Autodesk Inventor part; units mm, degrees
ref_plane "YZ Plane" through (0, 0, 0) normal (1, 0, 0) x (0, 1, 0)
ref_plane "XZ Plane" through (0, 0, 0) normal (0, 1, 0) x (-1, 0, 0)
ref_plane "XY Plane" through (0, 0, 0) normal (0, 0, 1) x (1, 0, 0)
sketch "Sketch2" plane through (0, 0, 0) normal (0, 1, 0) x (-1, 0, 0)
  line L0 (-22.05, -28.75) -> (22.05, -28.75)
  line L1 (22.05, -28.75) -> (22.05, 28.75)
  line L2 (22.05, 28.75) -> (-22.05, 28.75)
  line L3 (-22.05, 28.75) -> (-22.05, -28.75)
  line L4 (-22.05, -28.75) -> (22.05, 28.75) construction
  line L5 (22.05, -28.75) -> (-22.05, 28.75) construction
  point P0 (0, 0)
  dimension "d28" = 44.1
  dimension "d29" = 57.5
extrude "Extrusion2" add sketch "Sketch2" along normal blind 0.5
sketch "Sketch3" plane through (0, 0.5, 0) normal (0, 1, 0) x (1, 0, 0)
  line L0 (3.17, 0) -> (-3.4256, 0) construction
  line L1 (-18, -28.75) -> (-18, -19.75)
  line L2 (-15.5, -19.75) -> (-15.5, -28.75)
  arc A0 (-15.5, -19.75) -> (-18, -19.75) centre (-16.75, -19.75) ccw
  line L3 (-22.05, -28.75) -> (22.05, -28.75)
  line L4 (-22.05, 28.75) -> (-22.05, -28.75)
  line L5 (19.8, -28.75) -> (19.8, -19.75)
  line L6 (17.3, -19.75) -> (17.3, -28.75)
  arc A1 (19.8, -19.75) -> (17.3, -19.75) centre (18.55, -19.75) ccw
  line L7 (15.5, 28.75) -> (15.5, 19.75)
  line L8 (22.05, 28.75) -> (-22.05, 28.75)
  line L9 (18, 28.75) -> (18, 19.75)
  arc A2 (15.5, 19.75) -> (18, 19.75) centre (16.75, 19.75) ccw
  line L10 (22.05, -28.75) -> (22.05, 28.75)
  line L11 (-19.8, 28.75) -> (-19.8, 19.75)
  line L12 (-17.3, 28.75) -> (-17.3, 19.75)
  arc A3 (-19.8, 19.75) -> (-17.3, 19.75) centre (-18.55, 19.75) ccw
  point P0 (0, 0)
  point P1 (10.634, -28.75)
  point P2 (12.3949, -28.75)
  dimension "d32" = 2.5
  dimension "d33" = 9
  dimension "d34" = 1.25
  dimension "d48" = 5.3
  dimension "d60" = 9
  dimension "d61" = 9
  dimension "d62" = 1.25
  dimension "d64" = 9
  dimension "d65" = 9
  dimension "d66" = 1.25
  dimension "d71" = 3.5
  dimension "d87" = 5.3
  dimension "d88" = 3.5
extrude "Extrusion3" cut sketch "Sketch3" against normal through all contours L1 A0 L2 L3 | L6 A1 L5 L3 | L8 L12 A3 L11 | L8 L9 A2 L7
sketch "Sketch4" plane through (0, 0.5, 0) normal (0, 1, 0) x (1, 0, 0)
  line L0 (-22.05, 28.75) -> (-22.05, -28.75)
  line L1 (-22.05, -28.75) -> (22.05, -28.75)
  line L2 (22.05, -28.75) -> (22.05, 28.75)
  line L3 (22.05, 28.75) -> (-22.05, 28.75)
  point P0 (0, 0)
  point P1 (0, -27.15)
  point P2 (0, 27.15)
  point P3 (-18, -28.75)
  point P4 (-12.775, 28.75)
  dimension "d37" = 22.05
  dimension "d38" = 1.6
  dimension "d40" = 1.6
  dimension "d68" = 44.1
hole "Hole1" at (0, 0.5, 27.15) at (0, 0.5, -27.15) direction (0, -1, 0) diameter 2.4 end through all
sketch "Sketch5" plane through (0, 0.5, 0) normal (0, 1, 0) x (1, 0, 0)
  line L0 (-22.05, -28.75) -> (-18, -28.75)
  line L1 (-20.05, -28.75) -> (-22.05, -26.75)
  line L2 (-22.05, 28.75) -> (-22.05, -28.75)
  point P0 (0, 0)
  dimension "d49" = 2
  dimension "d50" = 2
extrude "Extrusion4" cut sketch "Sketch5" against normal through all
sketch "Sketch6" plane through (0, 0.5, 0) normal (0, 1, 0) x (1, 0, 0)
  circle A0 centre (0, -27.15) radius 1.2
  line L0 (-1.2, -27.15) -> (-1.2, -28.75)
  line L1 (-15.5, -28.75) -> (17.3, -28.75)
  line L2 (1.2, -27.15) -> (1.2, -28.75)
  line L3 (1.2, -27.15) -> (-1.2, -27.15)
  line L4 (24.0299, 0) -> (-42.1887, 0)
  line L5 (-1.2, 27.15) -> (-1.2, 28.75)
  line L6 (1.2, 27.15) -> (1.2, 28.75)
  line L7 (1.2, 27.15) -> (-1.2, 27.15)
  line L8 (15.5, 28.75) -> (-17.3, 28.75)
  point P0 (0, 0)
  point P1 (0, 27.15)
extrude "Extrusion5" cut sketch "Sketch6" against normal through all contours L2 L1 L0 A0 | L5 L8 L6 L7
sketch "Sketch7" plane through (0, 0.5, 0) normal (0, 1, 0) x (1, 0, 0)
  line L0 (-15.5, -19.75) -> (-15.5, -28.75)
  arc A0 (-18, -25.75) -> (-15.5, -25.75) centre (-16.75, -25.75) ccw
  line L1 (-18, -28.75) -> (-18, -19.75)
  arc A1 (-15.5, -19.75) -> (-18, -19.75) centre (-16.75, -19.75) ccw
  line L2 (-15.5, -28.75) -> (-1.2, -28.75)
  line L3 (-18, -28.75) -> (-15.5, -28.75)
  arc A2 (17.3, -25.75) -> (19.8, -25.75) centre (18.55, -25.75) ccw
  line L4 (17.3, -28.75) -> (17.3, -19.75)
  line L5 (19.8, -19.75) -> (19.8, -28.75)
  line L6 (1.2, -28.75) -> (17.3, -28.75)
  line L7 (17.3, -28.75) -> (19.8, -28.75)
  line L8 (-17.3, 28.75) -> (-17.3, 19.75)
  line L9 (-19.8, 19.75) -> (-19.8, 28.75)
  arc A3 (-17.3, 25.75) -> (-19.8, 25.75) centre (-18.55, 25.75) ccw
  line L10 (-1.2, 28.75) -> (-17.3, 28.75)
  line L11 (15.5, 28.75) -> (1.2, 28.75)
  arc A4 (18, 25.75) -> (15.5, 25.75) centre (16.75, 25.75) ccw
  line L12 (15.5, 19.75) -> (15.5, 28.75)
  line L13 (18, 28.75) -> (18, 19.75)
  line L14 (-19.8, 28.75) -> (-17.3, 28.75)
  line L15 (15.5, 28.75) -> (18, 28.75)
  point P0 (0, 0)
  dimension "d73" = 1.25
  dimension "d74" = 1.25
  dimension "d75" = 3
  dimension "d78" = 1.25
  dimension "d80" = 3
  dimension "d81" = 1.25
  dimension "d82" = 3
  dimension "d85" = 1.25
  dimension "d86" = 3
extrude "Extrusion6" add sketch "Sketch7" against normal up to surface (0.5 mm away) contours L0 L3 L1 A0 | A2 L5 L7 L4 | L8 A3 L9 L14 | A4 L12 L15 L13
equation "\"d34\" = 0.5 * d32"
equation "\"d60\" = d33"
equation "\"d61\" = d33"
equation "\"d62\" = d34"
equation "\"d64\" = d33"
equation "\"d65\" = d33"
equation "\"d66\" = d34"
equation "\"d87\" = d48"
equation "\"d88\" = d71"
equation "\"d73\" = d74"
equation "\"d78\" = d79"
equation "\"d80\" = d75"
equation "\"d81\" = d74"
equation "\"d82\" = d75"
equation "\"d85\" = d74"
equation "\"d86\" = d75"
properties part number "etl standard baseplate with cutouts"
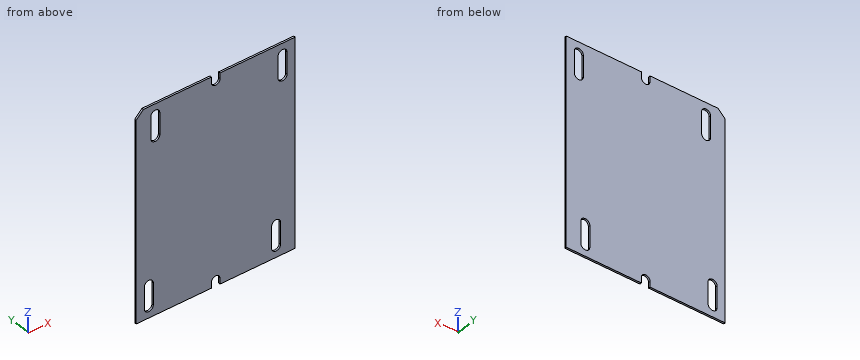
Part model, mm, in its own coordinate system. Round coordinates to 2 decimals unless told otherwise and drop trailing zeros. Loops run counter-clockwise (first coordinate to the right, second up) from the corner with the lowest first, then second, coordinate; pieces in that order, holes last.
Item 1: Cut at B-B, the plane z = -25. Give the cut face in (x, y), then the cut area to 4 significant figures.
Item 2: Drill centre lines: line 1 (X direction, y = 0.1, z = -20); line 2 (X direction, y = 0.45, z = 21); line 3 (Z direction, x = -17.5, y = 0.15). Where is each one in solid material? Low to high.
Item 3: Cut at C-C, the plane x = 0. Give the cut face in (y, z).
Item 4: Cut at A-A, the plane y = 0.3. State how many separate pieces and enclosed holes the cut face has, then the cut area to 3 significant figures.
A:
1. outline: (-22.05, 0) - (-19.8, 0) - (-19.8, 0.5) - (-22.05, 0.5) - close; (-17.3, 0) - (15.5, 0) - (15.5, 0.5) - (-17.3, 0.5) - close; (18, 0) - (22.05, 0) - (22.05, 0.5) - (18, 0.5) - close
1. area: 19.55 mm2
2. line 1: x = -22.05 to -19.8, -17.3 to 15.5, 18 to 22.05
2. line 2: x = -22.05 to -18, -15.5 to 17.3, 19.8 to 22.05
2. line 3: z = -28.75 to -26.43, -19.07 to 18.75, 26.75 to 28.75
3. outline: (0, -25.95) - (0.5, -25.95) - (0.5, 25.95) - (0, 25.95) - close
4. separate pieces: 1
4. enclosed holes: 4
4. area: 2,440 mm2
